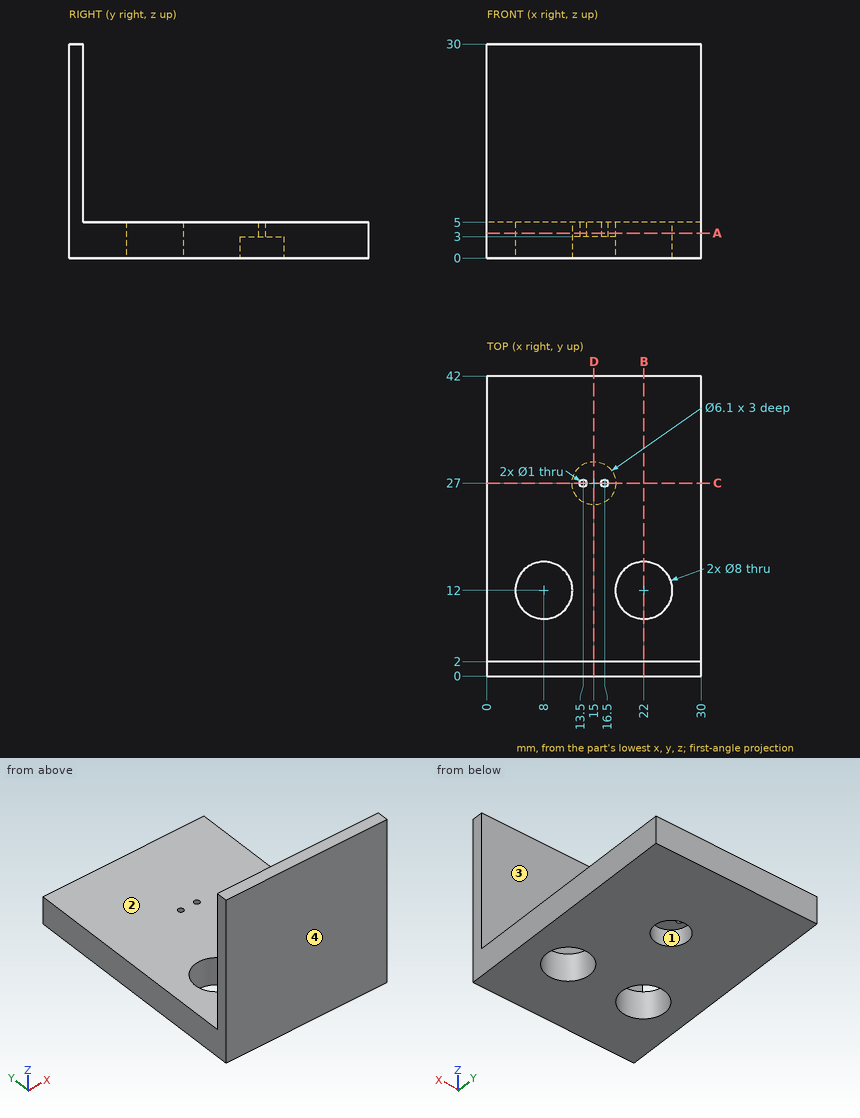
Print and shaded views of the part. All mm, measured from the part's lowest x, y and z. Give positions to 0.01 mm unless a question says otherwise; leave off trailing zeros. Loops run counter-clockwise (first coordinate to the right, second up) from the corner with the lowest first, then second, coordinate; pieces in that order, holes last. Notation, with made-up numbers: (29, 32.25) -> (83, 32.25) arc R20 ccw to (83, 46.25) -> close; hole circle Ø10 at (15, 16). An arc over 180 degrees is marked (long way). Answer in a Markdown table with one row per item.
Item 1: Slice it at D-D on x = 15. Write the cut outline in (y, z), plus the area to 3 significant figures.
Findings below:
| item | result |
|---|---|
| outline | (0, 0) -> (23.95, 0) -> (23.95, 3) -> (30.05, 3) -> (30.05, 0) -> (42, 0) -> (42, 5) -> (2, 5) -> (2, 30) -> (0, 30) -> close |
| area | 242 mm² |
Item 2: Slice it at A-A on z = 3.5. Write the cut outline in (x, y), plus the area to 3 significant figures.
Findings below:
| item | result |
|---|---|
| outline | (0, 0) -> (30, 0) -> (30, 42) -> (0, 42) -> close; hole circle Ø8 at (8, 12); hole circle Ø1 at (13.5, 27); hole circle Ø1 at (16.5, 27); hole circle Ø8 at (22, 12) |
| area | 1,160 mm² |
Item 3: Flat gauge pins, fed straight in: P1, Ø10, axis at x = 14.5, y = 21.5, coming from the +Z side; P2, Ø5, axis at x = 15, y = 27, coming from the -Z side; P3, Ø7, axis at x = 8, y = 12, coming from the +Z side; P4, Ø7.5, axis at x = 19, z = 16, coming from the +Y side. Where does each tip first touch, or does it go through?
Findings below:
| item | result |
|---|---|
| P1 | stops at z = 5 |
| P2 | stops at z = 3 |
| P3 | passes through |
| P4 | stops at y = 2 |
Item 4: Slice it at B-B on x = 22. Write the cut outline in (y, z).
Findings below:
| item | result |
|---|---|
| outline | (0, 0) -> (8, 0) -> (8, 5) -> (2, 5) -> (2, 30) -> (0, 30) -> close; (16, 0) -> (42, 0) -> (42, 5) -> (16, 5) -> close |
Item 5: Mould opens along Y. For the marked faces 1, 2, 3 and 4 say: pulls with the +Y half, pulls with the -Y half, needs draft (parallel to the pull), parting line crosses it, or undercut.
Findings below:
| item | result |
|---|---|
| face 1 | undercut |
| face 2 | needs draft |
| face 3 | pulls with the +Y half |
| face 4 | pulls with the -Y half |
Item 6: Slice it at C-C on y = 27. Write the cut outline in (x, z), plus the area to 3 significant figures.
Findings below:
| item | result |
|---|---|
| outline | (0, 0) -> (11.95, 0) -> (11.95, 3) -> (13, 3) -> (13, 5) -> (0, 5) -> close; (14, 3) -> (16, 3) -> (16, 5) -> (14, 5) -> close; (17, 3) -> (18.05, 3) -> (18.05, 0) -> (30, 0) -> (30, 5) -> (17, 5) -> close |
| area | 128 mm² |
Item 7: Probe line 1 along Y through (x, z) = (15, 1.5); line 2 along X through (y, z) = (27, 3.6); line 3 along Y through (x, z) = (16.5, 4.55). List the from-to ranges inside material, lowest first. Write a range as [from, to].
Findings below:
| item | result |
|---|---|
| line 1 | y = [0, 23.95], [30.05, 42] |
| line 2 | x = [0, 13], [14, 16], [17, 30] |
| line 3 | y = [0, 26.5], [27.5, 42] |
